from build123d import *

# Parameters (mm, degrees)
F1_DEPTH = 10
F2_R     = 2.49999


# Not quite as in the source:
# - a fillet or chamfer is up to 0.001 mm smaller than in the source, because OpenCascade refuses the exact size


with BuildPart() as f1:
    # F0 (on Top) → F1 (new body)
    with BuildSketch(Plane.XY):
        Polygon((-44.6886586582, 25.7738458982), (-44.6886586582, -29.2261541018), (-39.6886586582, -29.2261541018), (-39.6886586582, 20.7738458982), (30.3113413418, 20.7738458982), (30.3113413418, -29.2261541018), (35.3113413418, -29.2261541018), (35.3113413418, 25.7738458982), align=None)
    extrude(amount=F1_DEPTH)

    # F2 (radius 2.5 in the source; OpenCascade refuses exactly that, so slightly less here)
    f2_edges = [f1.edges().sort_by_distance(p)[0] for p in [
        (-44.688659, -1.726154, 10),
        (-39.688659, -4.226154, 10),
        (30.311341, -4.226154, 10),
        (35.311341, -1.726154, 10),
    ]]
    fillet(f2_edges, radius=F2_R)


solid = f1.part
Model file for the job. Use its own axes, mm. A direction names the side the tool comes from. Give positions to 0.01 mm unless a question says otherwise; leave off trailing zeros. Order: outer loops, then holes, each group sorted by start corner. A loop starts at its lowest first (then second) coordinate and runs counter-clockwise, first axis right, second up. Notation, with made-up numbers: (87, 42.5) - (105, 42.5) arc R18 cw to (105, 62.5) - close; hole circle Ø7 at (61.5, -31). An arc over 180 degrees is marked (long way). One line per item, written item: value.
Item 1: Slice it at B-B (z = 5.25). List the corners of the cut face in (x, y), then the cut area to 3 significant figures.
Response values:
outline: (-44.69, -29.23) - (-39.69, -29.23) - (-39.69, 20.77) - (30.31, 20.77) - (30.31, -29.23) - (35.31, -29.23) - (35.31, 25.77) - (-44.69, 25.77) - close
area: 900 mm2
Item 2: Tool access for faces 5 (the flat face through (-4, 25.774, 5)), 6 (the flat face through (-39.689, -5, 4)), 7 (the cylindrical face through (31.024, -4.576, 9.248)): list every direction of +Z, -Z, +X, -X, +Y, -Y with a clear straight run to the whole face (end or side of a thin tool).
Response values:
face 5: +Z, -Z, +X, -X, +Y
face 6: +Z, -Z, -Y
face 7: +Z, -Y
Item 3: Slice it at D-D (z = 9). List the corners of the cut face in (x, y).
Response values:
outline: (-44.19, -29.23) - (-40.19, -29.23) - (-40.19, 20.77) - (30.81, 20.77) - (30.81, -29.23) - (34.81, -29.23) - (34.81, 25.77) - (-44.19, 25.77) - close
Item 4: Two-plate mould, pull along X, no slides. Class faces 1 (the flat face through (-5, 23, 10)), 2 (the cylindrical face through (-40.402, -3.876, 9.248)), 3 (the flat face through (30.311, -4, 4)), 4 (the cylindrical face through (34.598, -1.341, 9.248)): released by +X, released by -X, zero draft, split by the parting line, or undercut.
Response values:
face 1: zero draft
face 2: undercut
face 3: undercut
face 4: released by +X
Item 5: Wall check: line 1 (X direction, y = -26, z = 3); line 2 (Y direction, x = 14.5, z = 3.75); line 3 (X direction, y = 7.5, z = 9.25). Give the ranges that are in metal, low to high.
Response values:
line 1: -44.69 to -39.69, 30.31 to 35.31
line 2: 20.77 to 25.77
line 3: -43.97 to -40.4, 31.03 to 34.6
Item 6: Slice it at C-C (x = 25). List the corners of the cut face in (y, z).
Response values:
outline: (20.77, 0) - (25.77, 0) - (25.77, 10) - (20.77, 10) - close
